Model file for the job. Use its own axes, mm. A direction names the side the tool comes from. Round coordinates to 2 decimals unless told otherwise and drop trailing zeros. Use a Markdown table: item, result.
from build123d import *

# Parameters (mm, degrees)
CROQUIS3_W                                  = 200
CROQUIS3_H                                  = 200
SALIENTE_EXTRUIR1_DEPTH                     = 10
CROQUIS4_W                                  = 72
CROQUIS4_H                                  = 102
CORTAR_EXTRUIR2_DEPTH                       = 5
CROQUIS5_W                                  = 5
CROQUIS5_H                                  = 70
CORTAR_EXTRUIR3_DEPTH                       = 142.774468788
REDONDEO1_R                                 = 10
REDONDEO2_R                                 = 10
REDONDEO3_R                                 = 10
REDONDEO4_R                                 = 10
REDONDEO5_R                                 = 10
REFRENTADO_PARA_TORNILLO_CON_CABEZA_2_COUNT = 2
REFRENTADO_PARA_TORNILLO_CON_CABEZA_2_PITCH = 180
REFRENTADO_PARA_TORNILLO_CON_CABEZA_3_COUNT = 2
REFRENTADO_PARA_TORNILLO_CON_CABEZA_3_PITCH = 254.558441227
REFRENTADO_PARA_TORNILLO_CON_CABEZA_4_COUNT = 2
REFRENTADO_PARA_TORNILLO_CON_CABEZA_4_PITCH = 180


# Some blends are built 0.0001 mm under size
with BuildPart() as part:
    # Croquis3 → Saliente-Extruir1 (new body)
    with BuildSketch(Plane.XY):
        Rectangle(CROQUIS3_W, CROQUIS3_H)
    extrude(amount=SALIENTE_EXTRUIR1_DEPTH)

    # Croquis4 → Cortar-Extruir2 (cut)
    with BuildSketch(Plane.XY.offset(10)):
        Rectangle(CROQUIS4_W, CROQUIS4_H)
    extrude(amount=-CORTAR_EXTRUIR2_DEPTH, mode=Mode.SUBTRACT)

    # Croquis5 → Cortar-Extruir3 (cut, through all)
    with BuildSketch(Plane.XY.offset(10)):
        Rectangle(CROQUIS5_W, CROQUIS5_H)
    extrude(amount=-CORTAR_EXTRUIR3_DEPTH, mode=Mode.SUBTRACT)

    # Redondeo1
    redondeo1_edges = [part.edges().sort_by_distance(p)[0] for p in [
        (-100, 0, 10),
        (0, -100, 10),
        (100, 0, 10),
        (0, 100, 10),
    ]]
    fillet(redondeo1_edges, radius=REDONDEO1_R - 0.0001)  # a hair under: the kernel refuses the full size

    # Redondeo2
    # the kernel refuses this fillet: 10 mm, written as the material it takes off along each edge
    with BuildSketch(Plane(origin=(90, 90, 10), x_dir=(1, 0, 0), z_dir=(0, -1, 0))) as redondeo2_piece_1:
        with BuildLine():
            CenterArc((0.0001, -9.9999), 9.9999, 0, 90)
            Line((10, -9.9999), (10, 0))
            Line((10, 0), (0.0001, 0))
        make_face()
    revolve(axis=Axis((90, 90, 10), (0, 0, 1)), revolution_arc=90, mode=Mode.SUBTRACT)
    with BuildSketch(Plane(origin=(100, 100, -25), x_dir=(0, -1, 0), z_dir=(0, 0, 1))) as redondeo2_piece_2:
        with BuildLine():
            CenterArc((REDONDEO2_R, -REDONDEO2_R), REDONDEO2_R, 90, 90)
            Line((0, -REDONDEO2_R), (0, 0))
            Line((0, 0), (REDONDEO2_R, 0))
        make_face()
    extrude(amount=35, mode=Mode.SUBTRACT)

    # Redondeo3
    # the kernel refuses this fillet: 10 mm, written as the material it takes off along each edge
    with BuildSketch(Plane(origin=(-90, -90, 10), x_dir=(-1, 0, 0), z_dir=(0, 1, 0))) as redondeo3_piece_1:
        with BuildLine():
            CenterArc((0.0001, -9.9999), 9.9999, 0, 90)
            Line((10, -9.9999), (10, 0))
            Line((10, 0), (0.0001, 0))
        make_face()
    revolve(axis=Axis((-90, -90, 10), (0, 0, 1)), revolution_arc=90, mode=Mode.SUBTRACT)
    with BuildSketch(Plane(origin=(-100, -100, -25), x_dir=(1, 0, 0), z_dir=(0, 0, 1))) as redondeo3_piece_2:
        with BuildLine():
            CenterArc((REDONDEO3_R, REDONDEO3_R), REDONDEO3_R, 180, 90)
            Line((0, REDONDEO3_R), (0, 0))
            Line((0, 0), (REDONDEO3_R, 0))
        make_face()
    extrude(amount=35, mode=Mode.SUBTRACT)

    # Redondeo4
    # the kernel refuses this fillet: 10 mm, written as the material it takes off along each edge
    with BuildSketch(Plane(origin=(90, -90, 10), x_dir=(0, -1, 0), z_dir=(-1, 0, 0))) as redondeo4_piece_1:
        with BuildLine():
            CenterArc((0.0001, -9.9999), 9.9999, 0, 90)
            Line((10, -9.9999), (10, 0))
            Line((10, 0), (0.0001, 0))
        make_face()
    revolve(axis=Axis((90, -90, 10), (0, 0, 1)), revolution_arc=90, mode=Mode.SUBTRACT)
    with BuildSketch(Plane(origin=(100, -100, -25), x_dir=(-1, 0, 0), z_dir=(0, 0, 1))) as redondeo4_piece_2:
        with BuildLine():
            CenterArc((REDONDEO4_R, -REDONDEO4_R), REDONDEO4_R, 90, 90)
            Line((0, -REDONDEO4_R), (0, 0))
            Line((0, 0), (REDONDEO4_R, 0))
        make_face()
    extrude(amount=35, mode=Mode.SUBTRACT)

    # Redondeo5
    # the kernel refuses this fillet: 10 mm, written as the material it takes off along each edge
    with BuildSketch(Plane(origin=(-90, 90, 10), x_dir=(0, 1, 0), z_dir=(1, 0, 0))) as redondeo5_piece_1:
        with BuildLine():
            CenterArc((0.0001, -9.9999), 9.9999, 0, 90)
            Line((10, -9.9999), (10, 0))
            Line((10, 0), (0.0001, 0))
        make_face()
    revolve(axis=Axis((-90, 90, 10), (0, 0, 1)), revolution_arc=90, mode=Mode.SUBTRACT)
    with BuildSketch(Plane(origin=(-100, 100, -25), x_dir=(0, -1, 0), z_dir=(0, 0, 1))) as redondeo5_piece_2:
        with BuildLine():
            CenterArc((REDONDEO5_R, REDONDEO5_R), REDONDEO5_R, 180, 90)
            Line((0, REDONDEO5_R), (0, 0))
            Line((0, 0), (REDONDEO5_R, 0))
        make_face()
    extrude(amount=35, mode=Mode.SUBTRACT)

    # Croquis16 → Refrentado para tornillo con cabeza troncocónica de #45 (revolve, cut)
    with BuildSketch(Plane(origin=(-90, 90, 10), x_dir=(0, -1, 0), z_dir=(1, 0, 0))):
        Polygon((0, 0), (0, 10), (1.63195, 10), (1.63195, 2.032), (3.175, 2.032), (3.175, 0.635), (3.81, 0), align=None)
    refrentado_para_tornillo_con_cabeza_tron = revolve(axis=Axis((-90, 90, 16.35), (0, 0, -1)), mode=Mode.SUBTRACT)

    # Refrentado para tornillo con cabeza  2: Refrentado para tornillo con cabeza troncocónica de #45 ×2
    with Locations(*[(i * REFRENTADO_PARA_TORNILLO_CON_CABEZA_2_PITCH, 0, 0) for i in range(1, REFRENTADO_PARA_TORNILLO_CON_CABEZA_2_COUNT)]):
        add(refrentado_para_tornillo_con_cabeza_tron, mode=Mode.SUBTRACT)

    # Refrentado para tornillo con cabeza  3: Refrentado para tornillo con cabeza troncocónica de #45 ×2
    with Locations(*[Vector(0.7071067811865476, -0.7071067811865476, 0) * (i * REFRENTADO_PARA_TORNILLO_CON_CABEZA_3_PITCH) for i in range(1, REFRENTADO_PARA_TORNILLO_CON_CABEZA_3_COUNT)]):
        add(refrentado_para_tornillo_con_cabeza_tron, mode=Mode.SUBTRACT)

    # Refrentado para tornillo con cabeza  4: Refrentado para tornillo con cabeza troncocónica de #45 ×2
    with Locations(*[(0, -i * REFRENTADO_PARA_TORNILLO_CON_CABEZA_4_PITCH, 0) for i in range(1, REFRENTADO_PARA_TORNILLO_CON_CABEZA_4_COUNT)]):
        add(refrentado_para_tornillo_con_cabeza_tron, mode=Mode.SUBTRACT)


solid = part.part
Q1. Pull direction X, two halves, no side cores. Call faces 4 (the face through (96.99, 1.26, 7.15)), 5 (the face through (-97.15, 1.26, 6.99)), 6 (the face through (87.23, 88.23, 9.48)): released by +X, released by -X, zero draft, split by the parting line, or undercut.
Results list:
| item | result |
|---|---|
| face 4 | released by +X |
| face 5 | released by -X |
| face 6 | undercut |
Q2. Drill centre lines: L1, parallel to X at y = -16, z = 1; L2, parallel to Y at x = -89, z = 7.75; L3, parallel to Y at x = -90, z = 9 (3 decimals). Where is each one in solid material? Low to high. Write a range as from..to.
Results list:
| item | result |
|---|---|
| L1 | x = -99.95..-2.5, 2.5..99.95 |
| L2 | y = -96.32..-91.29, -88.71..88.71, 91.29..96.32 |
| L3 | y = -94.359..-93.175, -86.825..86.825, 93.175..94.359 |
Q3. Flat gauge pins, fed straight in: pin 1 (4 mm diameter, centred on x = -90, y = 90, fed in from +Z); pin 2 (1.5 mm diameter, centred on y = 2, z = 8, fed in from -X); pin 3 (1 mm diameter, centred on x = 61, z = 1.5, fed in from +Y). Where does each tip first touch, or does it go through?
Results list:
| item | result |
|---|---|
| pin 1 | stops at z = 7.97 |
| pin 2 | stops at x = -96.89 |
| pin 3 | stops at y = 99.95 |
Q4. Tool access for faces 1 (the face through (1.26, 97.15, 6.99)), 2 (the face through (-90.95, -93.03, 8.68)), 3 (the face through (0, -35, 3)): list every direction of +Z, -Z, +X, -X, +Y, -Y with a clear straight run to the whole face (end or side of a thin tool).
Results list:
| item | result |
|---|---|
| face 1 | +Z, +X, -X, +Y |
| face 2 | +Z |
| face 3 | +Z, -Z |
Q5. Band-saw the part on D-D, the plane z = 2.75. Give the number of separate pieces and of enclosed holes in the cut face, plus the area to 3 significant figures.
Results list:
| item | result |
|---|---|
| separate pieces | 1 |
| enclosed holes | 5 |
| area | 39,200 mm² |
